from build123d import *

# Parameters (mm, degrees)
BOSS_EXTRUDE1_DEPTH      = 9
BOSS_EXTRUDE1_DEPTH_BACK = 6


with BuildPart() as part:
    # Sketch2 → Boss-Extrude1 (new, two sides)
    with BuildSketch(Plane.XY) as boss_extrude1_sk:
        with BuildLine():
            ThreePointArc((-1.285113167, -12.8458781), (-12.91, 0), (-1.285113167, 12.8458781))
            Line((-1.285113167, 12.8458781), (126.474646488, 25.627079044))
            ThreePointArc((126.474646488, 25.627079044), (154.793402461, 0), (126.474646488, -25.627079044))
            Line((126.474646488, -25.627079044), (-1.285113167, -12.8458781))
        make_face()
        with BuildLine():
            Line((-1.061139145, 10.607053489), (126.69862051, 23.388254433))
            ThreePointArc((126.69862051, 23.388254433), (152.543402461, 0), (126.69862051, -23.388254433))
            Line((126.69862051, -23.388254433), (-1.061139145, -10.607053489))
            ThreePointArc((-1.061139145, -10.607053489), (-10.66, 0), (-1.061139145, 10.607053489))
        make_face(mode=Mode.SUBTRACT)
    extrude(amount=BOSS_EXTRUDE1_DEPTH)
    extrude(boss_extrude1_sk.sketch, amount=-BOSS_EXTRUDE1_DEPTH_BACK)


solid = part.part
Can you work these out from the model? Positions are in its coordinate system, mm. A direction names the side the tool comes from. Round coordinates to 2 decimals unless told otherwise and drop trailing zeros. Loops run counter-clockwise (first coordinate to the right, second up) from the corner with the lowest first, then second, coordinate; pieces in that order, holes last. Notation, with made-up numbers: (-31, -10) - (-11, -10) arc R20 cw to (-11, 8) - close; hole circle Ø7 at (10, -15). An arc over 180 degrees is marked (long way). Answer in a Markdown table with one row per item. Add a question column.
Q1. I need wall thicknesses on L1, parallel to Y at x = 129, z = -4.75; L2, parallel to Y at x = 141, z = 5.75; L3, parallel to X at y = 3, z = 6. Which ranges of each line are inside material? Lowest first, please.
Q2. For pin 1 Ø2 at (y, z) = (-7, 3.5) entering from -X; pin 2 Ø6 at (x, z) = (14.5, -4.5) entering from -Y; pin 3 Ø1.5 at (y, z) = (-9.5, -4.5) entering from -X, each with a flat end and sliding along its axis, tell me the tip position at first contact or that it passes through.
Q3. Which directions (+Z, -Z, +X, -X, +Y, -Y) give clear straight access to the entire face, cutting with the end or side of a thin tool? Please do faces 1 (the flat face through (63.713, -17.087, 1.605)), 2 (the flat face through (61.7, 19.147, 1.605)).
Q4. I want a section at A-A on z = -3.25. List the corners of the cut face in (x, y) for me (3 decimals).
Q5. I want a section at C-C on x = 142. List the corners of the cut face in (y, z) for me, and give its area (3 significant figures).
Q6. I want a section at B-B on y = 0. List the corners of the cut face in (x, z) for me.
Q7. We'd pull the mould along X, two halves only. Please class faces 3 (the cylindrical face through (152.537, 0.55, 1.605)), 4 (the flat face through (78, 19, 9)), 5 (the flat face through (63.489, -19.326, 1.605)): pulls with the +X half, pulls with the -X half, needs draft (parallel to the pull), parting line crosses it, or undercut.
A:
| question | item | result |
|---|---|---|
| 1 | L1 | -25.75 to -23.5, 23.5 to 25.75 |
| 1 | L2 | -22.81 to -20.23, 20.23 to 22.81 |
| 1 | L3 | -12.56 to -10.23, 152.35 to 154.62 |
| 2 | pin 1 | x = -11.43 |
| 2 | pin 2 | y = -14.73 |
| 2 | pin 3 | x = -9.49 |
| 3 | face 1 | +Z, -Z |
| 3 | face 2 | +Z, -Z, -X, +Y |
| 4 | outline | (-1.285, -12.846) - (126.475, -25.627) arc R25.755 ccw (long way) to (126.475, 25.627) - (-1.285, 12.846) arc R12.91 ccw to start; hole (-1.061, -10.607) - (126.699, -23.388) arc R23.505 ccw (long way) to (126.699, 23.388) - (-1.061, 10.607) arc R10.66 ccw to start |
| 5 | outline | (-22.26, -6) - (-19.61, -6) - (-19.61, 9) - (-22.26, 9) - close; (19.61, -6) - (22.26, -6) - (22.26, 9) - (19.61, 9) - close |
| 5 | area | 79.4 mm^2 |
| 6 | outline | (-12.91, -6) - (-10.66, -6) - (-10.66, 9) - (-12.91, 9) - close; (152.54, -6) - (154.79, -6) - (154.79, 9) - (152.54, 9) - close |
| 7 | face 3 | undercut |
| 7 | face 4 | needs draft |
| 7 | face 5 | pulls with the -X half |
